Check sheet for the modelled part. Datum: model origin and axes. Units: mm. A direction names the side the tool comes from. Round coordinates to 2 decimals unless told otherwise and drop trailing zeros. Order: outer loops, then holes, each group sorted by start corner. A loop starts at its lowest first (then second) coordinate and runs counter-clockwise, first axis right, second up.
(1) Thickness scan on probe 1 along Y at (x, z) = (0, 15); probe 2 along Z at (x, y) = (-9.5, -13); probe 3 along X at (y, z) = (4, 15). Record the ranges inside material, lowest first.
(2) Depth check by flat-ended pin: pin 1 (6 mm diameter, centred on x = 7.5, z = 11.5, fed in from +Y); pin 2 (3 mm diameter, centred on x = 9, z = 2.5, fed in from -Y); pin 3 (8 mm diameter, centred on x = -10, z = 3.5, fed in from -Y). Enter the tip coordinate at first touch or a pass-through.
(3) Sectioned sample at A-A, the plane x = 0. Enter the section's corners in (y, z), and give its area (3 significant figures).
(4) Mould release check, pull along Y, two halves, no side actions. Record for faces 4 (the cylindrical face through (-17.204, 2.25, 20.254)), 5 (the flat face through (-9, 12, 20)), 6 (the flat face through (13.6, -2.4, 13.3)): released by +Y, released by -Y, zero draft, split by the parting line, or undercut.
(5) Sectioned sample at B-B, the plane z = 10.5. Enter the section's corners in (x, y).
(6) Tool access check on faces 1 (the flat face through (13.8, 0, 13.3)), 2 (the cylindrical face through (-12.394, 1.621, 9.614)), 3 (the cylindrical face through (-13.88, 1.82, 10.63)). Record the directions out of +Z, -Z, +X, -X, +Y, -Y that give a thin tool (end or side, any length) a straight path to the whole face; none if there is none.
```python
from build123d import *

# Parameters (mm, degrees)
F1_ANGLE = 350


with BuildPart() as f1:
    # F0 (on Front) → F1 (revolve)
    with BuildSketch(Plane.XZ):
        with BuildLine():
            Line((12.5, 19.5), (12.5, 0))
            Line((12.5, 0), (13.2, 0))
            Line((13.2, 0), (14, 1.5))
            Line((14, 1.5), (14, 19.5))
            ThreePointArc((14, 19.5), (14.146447, 19.853553), (14.5, 20))
            Line((14.5, 20), (17.35, 20))
            Line((17.35, 20), (17.35, 20.5))
            ThreePointArc((17.35, 20.5), (17.057107, 21.207107), (16.35, 21.5))
            Line((16.35, 21.5), (14.5, 21.5))
            ThreePointArc((14.5, 21.5), (13.085786, 20.914214), (12.5, 19.5))
        make_face()
    revolve(axis=Axis((0, 0, 24.386095), (0, 0, 1)), revolution_arc=F1_ANGLE)


solid = f1.part
```
Derived:
1. probe 1: y = -14 to -12.5, 12.5 to 14
1. probe 2: z = 20 to 21.5
1. probe 3: x = -13.42 to -11.84, 11.84 to 13.42
2. pin 1: stops at y = 13.26
2. pin 2: stops at y = -11.82
2. pin 3: stops at y = -12.65
3. outline: (-17.35, 20) - (-14.5, 20) arc R0.5 cw to (-14, 19.5) - (-14, 1.5) - (-13.2, 0) - (-12.5, 0) - (-12.5, 19.5) arc R2 ccw to (-14.5, 21.5) - (-16.35, 21.5) arc R1 ccw to (-17.35, 20.5) - close; (12.5, 0) - (13.2, 0) - (14, 1.5) - (14, 19.5) arc R0.5 cw to (14.5, 20) - (17.35, 20) - (17.35, 20.5) arc R1 ccw to (16.35, 21.5) - (14.5, 21.5) arc R2 ccw to (12.5, 19.5) - close
3. area: 71.3 mm2
4. face 4: split by the parting line
4. face 5: zero draft
4. face 6: undercut
5. outline: (12.31, -2.17) arc R12.5 cw (long way) to (12.5, 0) - (14, 0) arc R14 ccw (long way) to (13.79, -2.43) - close
6. face 1: +Z, -Z, +X
6. face 2: +Z, -Z
6. face 3: -Z
